```python
from build123d import *

# Parameters (mm, degrees)
SKETCH_1_W      = 240
SKETCH_1_H      = 40
EXTRUDE_1_DEPTH = 80
SKETCH_2_R      = 12
EXTRUDE_2_DEPTH = 15
SKETCH_3_R      = 12
EXTRUDE_3_DEPTH = 15


with BuildPart() as part:
    # 草图1 → 凸台-拉伸1 (new body)
    with BuildSketch(Plane.XY):
        with Locations((120, 20)):
            Rectangle(SKETCH_1_W, SKETCH_1_H)
    extrude(amount=EXTRUDE_1_DEPTH)

    # 草图2 → 凸台-拉伸2 (add)
    with BuildSketch(Plane(origin=(0, 0, 0), x_dir=(-1, 0, 0), z_dir=(0, 0, -1))):
        with Locations((-215, 20)):
            Circle(SKETCH_2_R)
        with Locations((-45, 20)):
            Circle(SKETCH_2_R)
    extrude(amount=EXTRUDE_2_DEPTH)

    # 草图3 → 凸台-拉伸3 (add)
    with BuildSketch(Plane.XY.offset(80)):
        with Locations(Location((25, 20, 0), (0, 0, 180))):
            Circle(SKETCH_3_R)
        with Locations(Location((195, 20, 0), (0, 0, 180))):
            Circle(SKETCH_3_R)
    extrude(amount=EXTRUDE_3_DEPTH)


solid = part.part
```
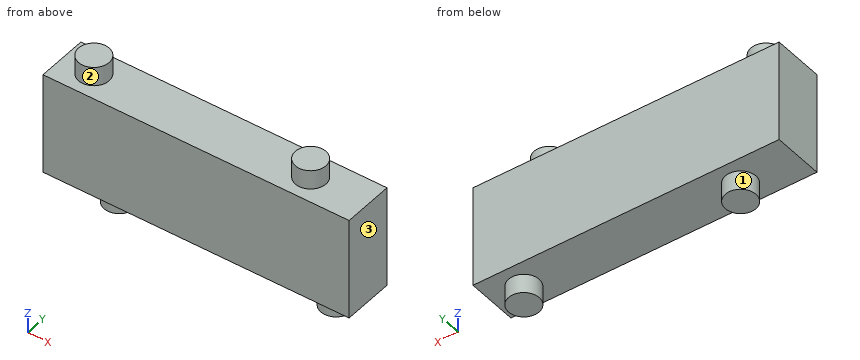
Input: part model. Units: mm. Frame: model coordinates. Face numbers are marked on the shaded views. A direction names the side the tool comes from. Round coordinates to 2 decimals unless told otherwise and drop trailing zeros. Loops run counter-clockwise (first coordinate to the right, second up) from the corner with the lowest first, then second, coordinate; pieces in that order, holes last.
1) Set-up query: the marked faces 1, 2 and 3. Return all of +Z, -Z, +X, -X, +Y, -Y with unobstructed straight access to the full face (end or side cutting, diameter ignored); none if empty.
Ans:
face 1: -Z
face 2: +Z
face 3: +Z, -Z, +X, +Y, -Y
2) Section query D-D on y = 5.5. Return the cut outline in (x, z), plus the area to 3 significant figures.
Ans:
outline: (0, 0) - (240, 0) - (240, 80) - (0, 80) - close
area: 19,200 mm2
3) Section query B-B on x = 25. Return the cut outline in (y, z), plus the area to 3 significant figures.
Ans:
outline: (0, 0) - (40, 0) - (40, 80) - (32, 80) - (32, 95) - (8, 95) - (8, 80) - (0, 80) - close
area: 3,560 mm2
4) Material intervals for line 1 (Z direction, x = 56, y = 17); line 2 (Z direction, x = 11, y = 31); line 3 (Y direction, x = 33.5, z = 87.5), sorted ascending.
Ans:
line 1: z = -15 to 80
line 2: z = 0 to 80
line 3: y = 11.53 to 28.47
5) Pin query (flat end, axial travel): pin 1 (20 mm diameter, centred on x = 95.5, y = 19, fed in from -Z); pin 2 (3 mm diameter, centred on x = 96.5, z = -2, fed in from +Y); pin 3 (5 mm diameter, centred on x = 76.5, y = 7, fed in from +Z). Return the tip coordinate at first contact, or that it passes through.
Ans:
pin 1: stops at z = 0
pin 2: passes through
pin 3: stops at z = 80
6) Section query C-C on x = 199.5. Return the cut outline in (y, z), plus the area to 3 significant figures.
Ans:
outline: (0, 0) - (40, 0) - (40, 80) - (31.12, 80) - (31.12, 95) - (8.88, 95) - (8.88, 80) - (0, 80) - close
area: 3,530 mm2
7) Section query A-A on y = 20. Return the cut outline in (x, z).
Ans:
outline: (0, 0) - (33, 0) - (33, -15) - (57, -15) - (57, 0) - (203, 0) - (203, -15) - (227, -15) - (227, 0) - (240, 0) - (240, 80) - (207, 80) - (207, 95) - (183, 95) - (183, 80) - (37, 80) - (37, 95) - (13, 95) - (13, 80) - (0, 80) - close
